For this review, use the dimensioned drawing (mm, ordinates from the lowest corner) and the shaded views. Round coordinates to 2 decimals unless told otherwise and drop trailing zeros. Write each loop counter-clockwise with the first axis right and the second up, starting at its lowest first coordinate (ties: lowest second). Pieces come first, ordered by that corner, then holes. Notation, with made-up numbers: (60.25, 74) -> (100.25, 74) arc R22 ccw to (100.25, 109) -> close; hole circle Ø10 at (74.25, 44). An arc over 180 degrees is marked (long way). Write each question's results on one line, items separated by ' | '. Start each with the question number.
Item 1: To check wall thickness, follow line 1 along X through (y, z) = (14, 6.35); line 2 along X through (y, z) = (25.4, 6.5); line 3 along Y through (x, z) = (19, 3.5). State the ranges of each line that lie inside material, in increasing order.
Item 2: Add section A-A (y = 25.4). Count the separate pieces of the cut face and the enclosed holes in it, plus the area to 3 significant figures.
Item 3: Clearance check with a flat-ended pin moving along its axis: pin 1 (1 mm diameter, centred on x = 30.5, y = 24, fed in from -Z). State where the tip first meets the part, or that it passes through.
Item 4: Add section B-B (x = 19.05). State the section outline as (y, z) points.
Item 5: The part is to be moulded in two halves that separate along Y. For the marked faces 1, 2, 3 and 4, say which applies: +Y half, -Y half, draft (parallel to the pull), parting line (faces both ways), or undercut.
Item 6: Add section D-D (x = 31.75). State the section outline as (y, z) points, plus the area to 3 significant figures.
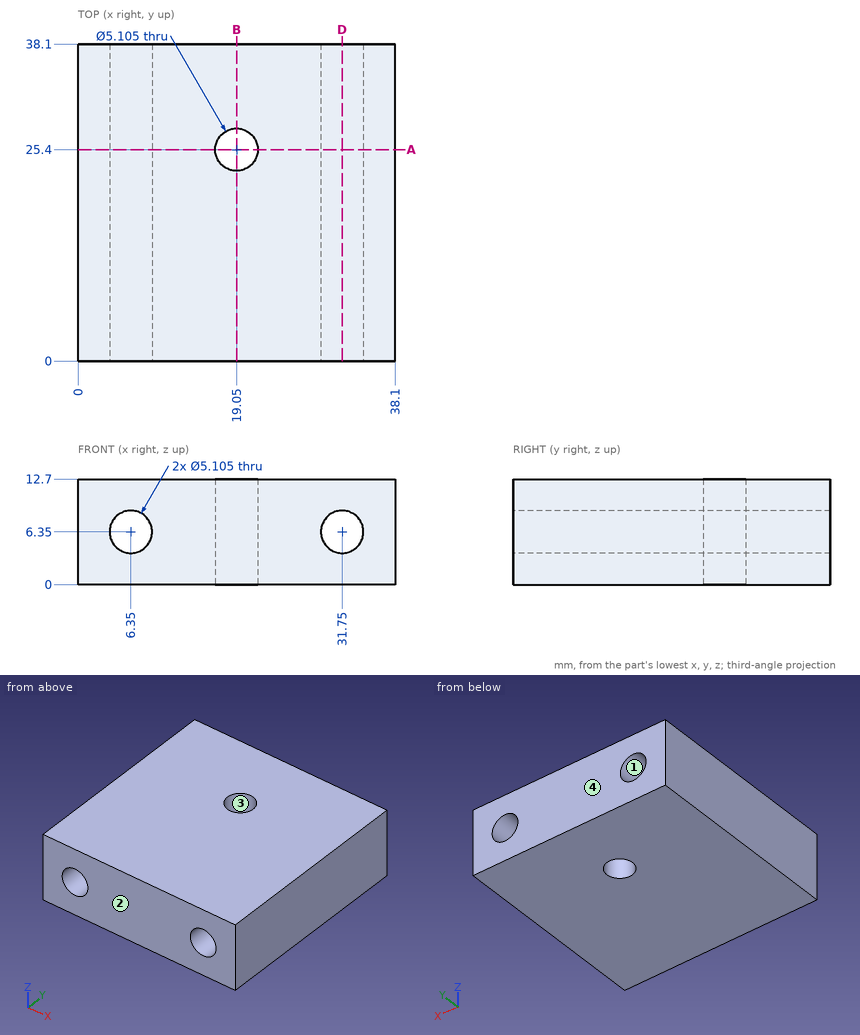
Responses:
1) line 1: x = 0 to 3.8, 8.9 to 29.2, 34.3 to 38.1 | line 2: x = 0 to 3.8, 8.9 to 16.5, 21.6 to 29.2, 34.3 to 38.1 | line 3: y = 0 to 22.85, 27.95 to 38.1
2) separate pieces: 2 | enclosed holes: 2 | area: 378 mm^2
3) pin 1: stops at z = 0
4) outline: (0, 0) -> (22.85, 0) -> (22.85, 12.7) -> (0, 12.7) -> close; (27.95, 0) -> (38.1, 0) -> (38.1, 12.7) -> (27.95, 12.7) -> close
5) face 1: draft | face 2: -Y half | face 3: undercut | face 4: +Y half
6) outline: (0, 0) -> (38.1, 0) -> (38.1, 3.8) -> (0, 3.8) -> close; (0, 8.9) -> (38.1, 8.9) -> (38.1, 12.7) -> (0, 12.7) -> close | area: 289 mm^2
